Here's the drawing with two shaded views (mm, measured from the low corner). I have some questions. Round coordinates to 2 decimals unless told otherwise and drop trailing zeros. Order: outer loops, then holes, each group sorted by start corner. A loop starts at its lowest first (then second) coordinate and runs counter-clockwise, first axis right, second up.
Q1. If we section it at C-C (y = 3.75): Please give me the cut outline in (x, z).
Q2. If we section it at D-D (x = 5.25): Please give me the cut outline in (y, z).
Q3. We'd pull the mould along X, two halves only. Please class the marked faces 1, 2 and 3: pulls with the +X half, pulls with the -X half, needs draft (parallel to the pull), parting line crosses it, or undercut.
Q4. If we section it at B-B (x = 2.25): Please give me the cut outline in (y, z).
Q5. Will this pin go through, and if not, where does the flat tip stop? P1, Ø1.5, axis at y = 1.5, z = 7, coming from the +X side.
Q6. If I drill on line 1 (Y direction, x = 2.5, z = 11.25); line 2 (X direction, y = 3.3, z = 1.75); line 3 (X direction, y = 3.95, z = 17) (1 decimal), over which ranges is the centre line in solid material (lowest first)?
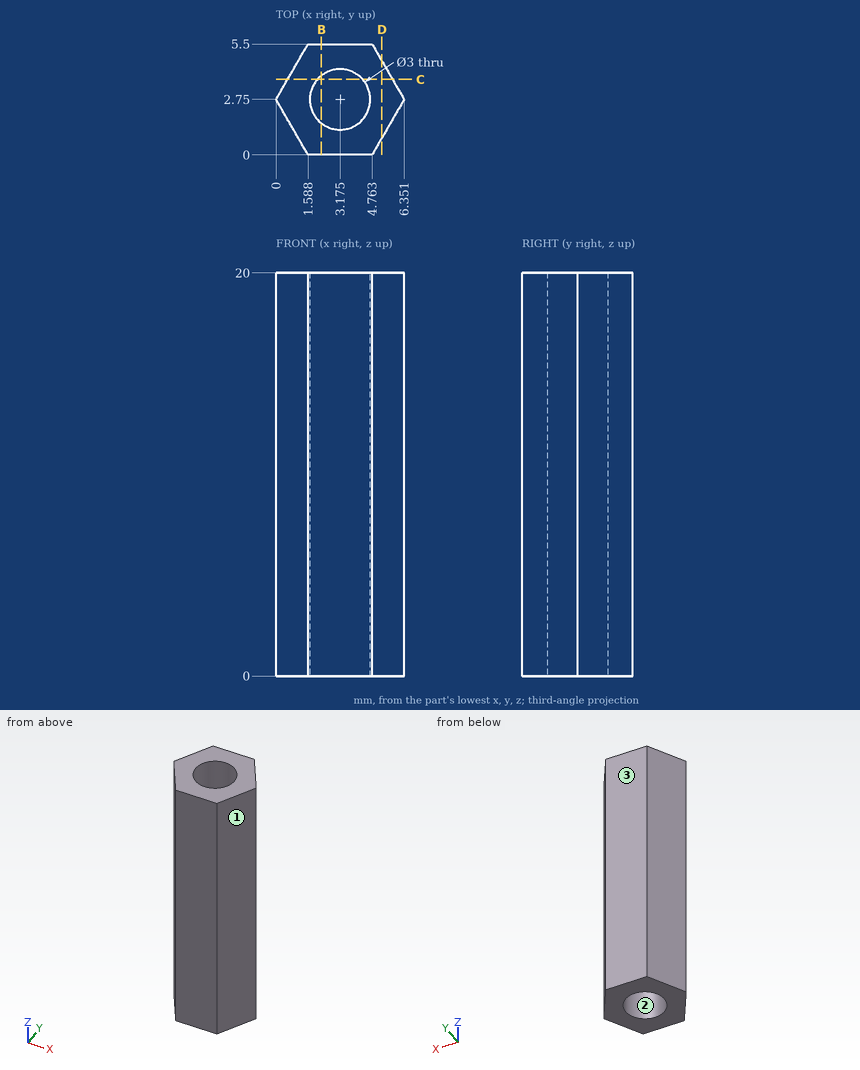
Solution:
1. outline: (0.58, 0) - (2.06, 0) - (2.06, 20) - (0.58, 20) - close; (4.29, 0) - (5.77, 0) - (5.77, 20) - (4.29, 20) - close
2. outline: (0.84, 0) - (4.66, 0) - (4.66, 20) - (0.84, 20) - close
3. face 1: pulls with the +X half
3. face 2: undercut
3. face 3: needs draft
4. outline: (0, 0) - (1.57, 0) - (1.57, 20) - (0, 20) - close; (3.93, 0) - (5.5, 0) - (5.5, 20) - (3.93, 20) - close
5. P1: stops at x = 6.06
6. line 1: y = 0 to 1.41, 4.09 to 5.5
6. line 2: x = 0.32 to 1.78, 4.57 to 6.03
6. line 3: x = 0.7 to 2.3, 4.1 to 5.7
